Geometry check sheet. Reference: the model listing, model coordinates, mm. A direction names the side the tool comes from. Round coordinates to 2 decimals unless told otherwise and drop trailing zeros. Write each loop counter-clockwise with the first axis right and the second up, starting at its lowest first coordinate (ties: lowest second). Pieces come first, ordered by that corner, then holes.
Item 1: Scan lines: probe 1 along Y at (x, z) = (-38.5, 68); probe 2 along X at (y, z) = (43.5, 19); probe 3 along X at (y, z) = (26, 80.5). Record each from-to range of solid material in increasing order.
Item 2: Draft check along X on faces 4 (the face through (-114.884, 50, 61)), 5 (the face through (-256.824, 100.783, 61.108)), 6 (the face through (-113, -19, 0)). Enter one of: pulls with the +X half, pulls with the -X half, needs draft (parallel to the pull), parting line crosses it, or undercut.
Item 3: Access from +Z, -Z, +X, -X, +Y, -Y to the whole of each face (thin tool, end or side, straight path). Record for faces 1 (the face through (17, -62.583, 61)), 2 (the face through (20, 64.165, 61)), 3 (the face through (151.267, 0, 61)).
Item 4: Depth check by flat-ended pin: P1, Ø4, axis at x = -60, z = 95, coming from the -Y side; P2, Ø2, axis at x = -275.5, z = 72, coming from the +Y side; P3, Ø8.5, axis at y = 52.5, z = 44, coming from the -X side. Enter the tip coordinate at first touch or a pass-through.
Item 5: Cross-section at A-A (z = 88.5). Enter the section's corners in (x, y), then the cut area to 3 significant figures.
Item 6: Cross-section at C-C (y = -114). Enter the section's corners in (x, z), then the cut area to 3 significant figures.
Item 7: Cross-section at B-B (x = -299). Enter the section's corners in (y, z), then the cut area to 3 significant figures.
from build123d import *

# Parameters (mm, degrees)
BOSS_EXTRUDE1_DEPTH = 123.952


with BuildPart() as part:
    # Sketch1 → Boss-Extrude1 (new body)
    with BuildSketch(Plane.XY):
        with BuildLine():
            ThreePointArc((-150.141788754, -129.869756414), (-205.816359245, -15.653721009), (-181.433254288, 109.047621148))
            Line((-181.433254288, 109.047621148), (-187.831275189, 116.037713042))
            Line((-187.831275189, 116.037713042), (-327.77572694, 85.095221198))
            Line((-327.77572694, 85.095221198), (-370.950968822, -51.57147506))
            Line((-370.950968822, -51.57147506), (-274.181758953, -157.295679473))
            Line((-274.181758953, -157.295679473), (-150.141788754, -129.869756414))
        make_face()
        Polygon((151.2671863, 64.164969875), (-114.883967634, 64.164969875), (-114.883967634, 36.339882858), (-91.062065319, 10.313508629), (-114.09129189, -62.583090802), (151.2671863, -62.583090802), align=None)
        Polygon((-91.062065319, 10.313508629), (-114.883967634, 36.339882858), (-114.883967634, -62.583090802), (-114.09129189, -62.583090802), align=None)
        with BuildLine():
            Line((-114.883967634, -62.583090802), (-114.883967634, 36.339882858))
            Line((-114.883967634, 36.339882858), (-181.433254288, 109.047621148))
            ThreePointArc((-181.433254288, 109.047621148), (-205.816359245, -15.653721009), (-150.141788754, -129.869756414))
            Line((-150.141788754, -129.869756414), (-134.237307201, -126.353187629))
            Line((-134.237307201, -126.353187629), (-114.09129189, -62.583090802))
            Line((-114.09129189, -62.583090802), (-114.883967634, -62.583090802))
        make_face()
    extrude(amount=BOSS_EXTRUDE1_DEPTH)


solid = part.part
Resolved:
1. probe 1: y = -62.58 to 64.16
1. probe 2: x = -340.92 to -121.44, -114.88 to 151.27
1. probe 3: x = -346.44 to 151.27
2. face 4: undercut
2. face 5: pulls with the -X half
2. face 6: needs draft
3. face 1: +Z, -Z, +X, -Y
3. face 2: +Z, -Z, +X, +Y
3. face 3: +Z, -Z, +X, +Y, -Y
4. P1: stops at y = -62.58
4. P2: stops at y = 96.87
4. P3: stops at x = -339.42
5. outline: (-370.95, -51.57) - (-274.18, -157.3) - (-134.24, -126.35) - (-114.09, -62.58) - (151.27, -62.58) - (151.27, 64.16) - (-114.88, 64.16) - (-114.88, 36.34) - (-187.83, 116.04) - (-327.78, 85.1) - close
5. area: 85,900 mm2
6. outline: (-313.81, 0) - (-130.33, 0) - (-130.33, 123.95) - (-313.81, 123.95) - close
6. area: 22,700 mm2
7. outline: (-130.18, 0) - (91.46, 0) - (91.46, 123.95) - (-130.18, 123.95) - close
7. area: 27,500 mm2
